Part model, mm, in its own coordinate system. Give positions to 0.01 mm unless a question says otherwise; leave off trailing zeros. Order: outer loops, then holes, each group sorted by start corner. A loop starts at its lowest first (then second) coordinate and runs counter-clockwise, first axis right, second up. Notation, with made-up numbers: (24.25, 71) -> (63.25, 71) arc R20 ccw to (63.25, 96) -> close; hole circle Ø3 at (81.5, 44). An arc over 180 degrees is marked (long way). Write item = value, one per line. Start each with the question number.
Item 1: Band-saw the part on B-B on z = 12.5. Write the cut outline in (x, y), plus the area to 3 significant figures.
Item 2: Flat gauge pin, fed straight in: P1, Ø4.5, axis at x = 51, z = 0, coming from the -Y side. Where does the tip first touch, or does it go through?
Item 3: Band-saw the part on C-C on x = 11. Write the cut outline in (y, z), plus the area to 3 significant figures.
Item 4: Drill centre lines: line 1 along X through (y, z) = (2.6, -32); line 2 along Z through (x, y) = (-51, 2.25). Where is each one in solid material? Low to high.
Item 5: Band-saw the part on A-A on y = 1.9. Write the cut outline in (x, z), plus the area to 3 significant figures.
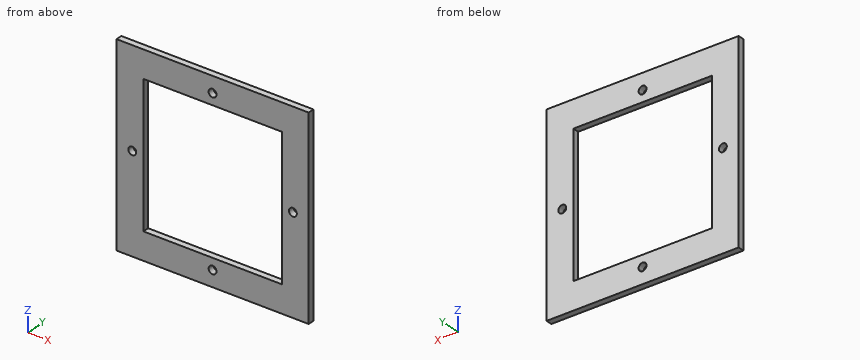
```python
from build123d import *

# Parameters (mm, degrees)
BOSS_EXTRUDE1_DEPTH = 4


with BuildPart() as part:
    # Sketch1 → Boss-Extrude1 (new body)
    with BuildSketch(Plane(origin=(0, 0, 0), x_dir=(1, 0, 0), z_dir=(0, 1, 0))):
        with BuildLine():
            Line((-61, -61), (0, -61))
            Line((0, -61), (0, -53.5))
            ThreePointArc((0, -53.5), (-2.5, -51), (0, -48.5))
            Line((0, -48.5), (0, -44))
            Line((0, -44), (-44, -44))
            Line((-44, -44), (-44, 0))
            Line((-44, 0), (-48.5, 0))
            ThreePointArc((-48.5, 0), (-51, -2.5), (-53.5, 0))
            Line((-53.5, 0), (-61, 0))
            Line((-61, 0), (-61, -61))
        make_face()
        with BuildLine():
            Line((61, 0), (53.5, 0))
            ThreePointArc((53.5, 0), (51, -2.5), (48.5, 0))
            Line((48.5, 0), (44, 0))
            Line((44, 0), (44, -44))
            Line((44, -44), (0, -44))
            Line((0, -44), (0, -48.5))
            ThreePointArc((0, -48.5), (1.767766953, -49.232233047), (2.5, -51))
            ThreePointArc((2.5, -51), (1.767766953, -52.767766953), (0, -53.5))
            Line((0, -53.5), (0, -61))
            Line((0, -61), (61, -61))
            Line((61, -61), (61, 0))
        make_face()
        with BuildLine():
            ThreePointArc((48.5, 0), (51, 2.5), (53.5, 0))
            Line((53.5, 0), (61, 0))
            Line((61, 0), (61, 61))
            Line((61, 61), (0, 61))
            Line((0, 61), (0, 53.5))
            ThreePointArc((0, 53.5), (1.767766953, 52.767766953), (2.5, 51))
            ThreePointArc((2.5, 51), (1.767766953, 49.232233047), (0, 48.5))
            Line((0, 48.5), (0, 44))
            Line((0, 44), (44, 44))
            Line((44, 44), (44, 0))
            Line((44, 0), (48.5, 0))
        make_face()
        with BuildLine():
            Line((0, 53.5), (0, 61))
            Line((0, 61), (-61, 61))
            Line((-61, 61), (-61, 0))
            Line((-61, 0), (-53.5, 0))
            ThreePointArc((-53.5, 0), (-51, 2.5), (-48.5, 0))
            Line((-48.5, 0), (-44, 0))
            Line((-44, 0), (-44, 44))
            Line((-44, 44), (0, 44))
            Line((0, 44), (0, 48.5))
            ThreePointArc((0, 48.5), (-2.5, 51), (0, 53.5))
        make_face()
    extrude(amount=BOSS_EXTRUDE1_DEPTH)


solid = part.part
```
Values found:
q1.outline = (-61, 0) -> (-44, 0) -> (-44, 4) -> (-61, 4) -> close; (44, 0) -> (61, 0) -> (61, 4) -> (44, 4) -> close
q1.area = 136 mm^2
q2.P1 = through
q3.outline = (0, -61) -> (4, -61) -> (4, -44) -> (0, -44) -> close; (0, 44) -> (4, 44) -> (4, 61) -> (0, 61) -> close
q3.area = 136 mm^2
q4.line_1 = -61 to -44, 44 to 61
q4.line_2 = -61 to -2.5, 2.5 to 61
q5.outline = (-61, -61) -> (61, -61) -> (61, 61) -> (-61, 61) -> close; hole circle Ø5 at (-51, 0); hole (-44, -44) -> (44, -44) -> (44, 44) -> (-44, 44) -> close; hole circle Ø5 at (0, -51); hole circle Ø5 at (0, 51); hole circle Ø5 at (51, 0)
q5.area = 7,060 mm^2
